Model file for the job. Use its own axes, mm. A direction names the side the tool comes from. Give positions to 0.01 mm unless a question says otherwise; leave off trailing zeros. Write each loop counter-clockwise with the first axis right and the second up, starting at its lowest first coordinate (ties: lowest second). Pieces come first, ordered by that corner, then holes. Notation, with made-up numbers: M -17.5,-24.5 L 31.5,-24.5 A29 ccw 31.5,6.5 Z; hole C 81,36 d1. An arc over 180 degrees is marked long. Answer as a JSON object with one key per item and string values. Group by question number.
```python
from build123d import *

# Parameters (mm, degrees)
SKETCH1_W           = 40.5
SKETCH1_H           = 40.5
BOSS_EXTRUDE1_DEPTH = 4.8
SKETCH2_R           = 8.5
BOSS_EXTRUDE2_DEPTH = 3.5
SKETCH3_R           = 1.5
CUT_EXTRUDE1_DEPTH  = 4.8
SKETCH4_R           = 20.25
BOSS_EXTRUDE3_DEPTH = 1.5


with BuildPart() as part:
    # Sketch1 → Boss-Extrude1 (new body)
    with BuildSketch(Plane(origin=(0, 0, 0), x_dir=(1, 0, 0), z_dir=(0, 1, 0))):
        Rectangle(SKETCH1_W, SKETCH1_H)
    extrude(amount=BOSS_EXTRUDE1_DEPTH)

    # Sketch2 → Boss-Extrude2 (add)
    with BuildSketch(Plane(origin=(0, 4.8, 0), x_dir=(1, 0, 0), z_dir=(0, 1, 0))):
        Circle(SKETCH2_R)
    extrude(amount=BOSS_EXTRUDE2_DEPTH)

    # Sketch3 → Cut-Extrude1 (cut)
    with BuildSketch(Plane(origin=(0, 4.8, 0), x_dir=(1, 0, 0), z_dir=(0, 1, 0))):
        with Locations((17, 17)):
            Circle(SKETCH3_R)
        with Locations((-17, 17)):
            Circle(SKETCH3_R)
        with Locations((-17, -17)):
            Circle(SKETCH3_R)
        with Locations((17, -17)):
            Circle(SKETCH3_R)
    extrude(amount=-CUT_EXTRUDE1_DEPTH, mode=Mode.SUBTRACT)

    # Sketch4 → Boss-Extrude3 (add)
    with BuildSketch(Plane(origin=(0, 0, 0), x_dir=(-1, 0, 0), z_dir=(0, -1, 0))):
        Circle(SKETCH4_R)
    extrude(amount=BOSS_EXTRUDE3_DEPTH)


solid = part.part
```
Q1. Slice it at A-A, the plane y = 3.75. Write the cut outline in (x, z), then the cut area to 3 significant figures.
Q2. Two-plate mould, pull along X, no slides. Class faces 1 (the flat face through (-15, 0, -15)), 2 (the cylindrical face through (15.89, 2.43, -18.01)), 3 (the cylindrical face through (4.57, 6.526, -7.167)): +X half, -X half, draft (parallel to the pull), parting line (faces both ways), or undercut.
Q3. Wall check: L1, parallel to Z at x = -17, y = 2.9; L2, parallel to X at y = 4, z = 16. Give the ranges that are in metal, low to high.
Q4. 3-axis set-ups, long thin cutter, end or side, ignore diameter. For faces 4 (the flat face through (15, 0, 15)), 5 (the cylindrical face through (-11, -1, -17)), 6 (the flat face through (-15, 0, 16)), 7 (the flat face through (-9, 4.8, 0)): which of +Z, -Z, +X, -X, +Y, -Y reach the whole face in a straight line?
Q5. Slice it at C-C, the plane x = 17. Write the cut outline in (y, z), then the cut area to 3 significant figures.
Q6. Slice it at B-B, the plane z = -17. Write the cut outline in (x, y), then the cut area to 3 significant figures.
Q7. Slice it at D-D, the plane x = 5. Write the cut outline in (y, z).
Q8. Drop flat-ended pins along their axis: P1, Ø4, axis at x = 9, z = 12.5, coming from the +Y side; P2, Ø1.8, axis at x = 17, z = 17, coming from the +Y side. Give the stop position or say it passes through.
Solved:
{
 "1": {"outline": "M -20.25,-20.25 L 20.25,-20.25 L 20.25,20.25 L -20.25,20.25 Z; hole C -17,-17 d3; hole C -17,17 d3; hole C 17,-17 d3; hole C 17,17 d3", "area": "1,610 mm²"},
 "2": {"face 1": "draft", "face 2": "undercut", "face 3": "parting line"},
 "3": {"L1": "z = -20.25 to -18.5, -15.5 to 15.5, 18.5 to 20.25", "L2": "x = -20.25 to -18.12, -15.88 to 15.88, 18.12 to 20.25"},
 "4": {"face 4": "+Z, +X, -Y", "face 5": "-Y", "face 6": "+Z, -X, -Y", "face 7": "+Y"},
 "5": {"outline": "M -1.5,-11 L 0,-11 L 0,-15.5 L 4.8,-15.5 L 4.8,15.5 L 0,15.5 L 0,11 L -1.5,11 Z; M 0,-20.25 L 4.8,-20.25 L 4.8,-18.5 L 0,-18.5 Z; M 0,18.5 L 4.8,18.5 L 4.8,20.25 L 0,20.25 Z", "area": "199 mm²"},
 "6": {"outline": "M -20.25,0 L -18.5,0 L -18.5,4.8 L -20.25,4.8 Z; M -15.5,0 L -11,0 L -11,-1.5 L 11,-1.5 L 11,0 L 15.5,0 L 15.5,4.8 L -15.5,4.8 Z; M 18.5,0 L 20.25,0 L 20.25,4.8 L 18.5,4.8 Z", "area": "199 mm²"},
 "7": {"outline": "M -1.5,-19.62 L 0,-19.62 L 0,-20.25 L 4.8,-20.25 L 4.8,-6.87 L 8.3,-6.87 L 8.3,6.87 L 4.8,6.87 L 4.8,20.25 L 0,20.25 L 0,19.62 L -1.5,19.62 Z"},
 "8": {"P1": "stops at y = 4.8", "P2": "passes through"}
}
